```python
from build123d import *

# Parameters (mm, degrees)
SKETCH_22_W         = 80
SKETCH_22_H         = 80
SKETCH_22_R         = 1.6
SKETCH_22_R_2       = 23.7
SKETCH_22_R_3       = 2.6
EXTRUDE_1_DEPTH     = 15
SKETCH_24_R         = 2.9
CUT_EXTRUDE_2_DEPTH = 5
SKETCH_26_R         = 4.5
CUT_EXTRUDE_4_DEPTH = 5
SKETCH_31_R         = 1.8
CUT_EXTRUDE_6_DEPTH = 12
SKETCH_36_R         = 1.8
CUT_EXTRUDE_9_DEPTH = 12


with BuildPart() as part:
    # 草图22 → 凸台-拉伸1 (new body)
    with BuildSketch(Plane(origin=(0, 0, 0), x_dir=(1, 0, 0), z_dir=(0, 1, 0))):
        Rectangle(SKETCH_22_W, SKETCH_22_H)
        with Locations((0, 37)):
            Circle(SKETCH_22_R, mode=Mode.SUBTRACT)
        with Locations((26.162950904, 26.162950904)):
            Circle(SKETCH_22_R, mode=Mode.SUBTRACT)
        with Locations((37, 0)):
            Circle(SKETCH_22_R, mode=Mode.SUBTRACT)
        with Locations((26.162950904, -26.162950904)):
            Circle(SKETCH_22_R, mode=Mode.SUBTRACT)
        with Locations((0, -37)):
            Circle(SKETCH_22_R, mode=Mode.SUBTRACT)
        with Locations((-26.162950904, -26.162950904)):
            Circle(SKETCH_22_R, mode=Mode.SUBTRACT)
        with Locations((-37, 0)):
            Circle(SKETCH_22_R, mode=Mode.SUBTRACT)
        with Locations((-26.162950904, 26.162950904)):
            Circle(SKETCH_22_R, mode=Mode.SUBTRACT)
        Circle(SKETCH_22_R_2, mode=Mode.SUBTRACT)
        with Locations((-31.819805153, 31.819805153)):
            Circle(SKETCH_22_R_3, mode=Mode.SUBTRACT)
        with Locations((-31.819805153, -31.819805153)):
            Circle(SKETCH_22_R_3, mode=Mode.SUBTRACT)
        with Locations((31.819805153, -31.819805153)):
            Circle(SKETCH_22_R_3, mode=Mode.SUBTRACT)
        with Locations((31.819805153, 31.819805153)):
            Circle(SKETCH_22_R_3, mode=Mode.SUBTRACT)
    extrude(amount=EXTRUDE_1_DEPTH)

    # 草图24 → 切除-拉伸2 (cut)
    with BuildSketch(Plane.XZ):
        with Locations((0, 37)):
            Circle(SKETCH_24_R)
        with Locations((26.162950904, 26.162950904)):
            Circle(SKETCH_24_R)
        with Locations((37, 0)):
            Circle(SKETCH_24_R)
        with Locations((26.162950904, -26.162950904)):
            Circle(SKETCH_24_R)
        with Locations((0, -37)):
            Circle(SKETCH_24_R)
        with Locations((-26.162950904, -26.162950904)):
            Circle(SKETCH_24_R)
        with Locations((-37, 0)):
            Circle(SKETCH_24_R)
        with Locations((-26.162950904, 26.162950904)):
            Circle(SKETCH_24_R)
    extrude(amount=-CUT_EXTRUDE_2_DEPTH, mode=Mode.SUBTRACT)

    # 草图26 → 切除-拉伸4 (cut)
    with BuildSketch(Plane(origin=(0, 15, 0), x_dir=(1, 0, 0), z_dir=(0, 1, 0))):
        with Locations((-31.819805153, 31.819805153)):
            Circle(SKETCH_26_R)
        with Locations((31.819805153, 31.819805153)):
            Circle(SKETCH_26_R)
        with Locations((31.819805153, -31.819805153)):
            Circle(SKETCH_26_R)
        with Locations((-31.819805153, -31.819805153)):
            Circle(SKETCH_26_R)
    extrude(amount=-CUT_EXTRUDE_4_DEPTH, mode=Mode.SUBTRACT)

    # 草图31 → 切除-拉伸6 (cut)
    with BuildSketch(Plane.XY.offset(40)):
        with Locations((13.998307963, 7.310553575)):
            Circle(SKETCH_31_R)
    extrude(amount=-CUT_EXTRUDE_6_DEPTH, mode=Mode.SUBTRACT)

    # 草图36 → 切除-拉伸9 (cut)
    with BuildSketch(Plane(origin=(0, 0, -40), x_dir=(-1, 0, 0), z_dir=(0, 0, -1))):
        with Locations((-16.504769552, 7.351157317)):
            Circle(SKETCH_36_R)
    extrude(amount=-CUT_EXTRUDE_9_DEPTH, mode=Mode.SUBTRACT)


solid = part.part
```
Could you check a few things on this model? Use its own coordinates, in mm. A direction names the side the tool comes from. Coordinates: 2 decimals unless noted, no trailing zeros. Order: outer loops, then holes, each group sorted by start corner. A loop starts at its lowest first (then second) coordinate and runs counter-clockwise, first axis right, second up. Notation, with made-up numbers: M 55,-35.5 L 61,-35.5 A21 cw 61,-16.5 Z; hole C -26.75,52 d7. An arc over 180 degrees is marked long. Use a Markdown table: item, result. Add a question column.
Q1. Which directions (+Z, -Z, +X, -X, +Y, -Y) give clear straight access to the entire face, cutting with the end or side of a thin tool? Please do faces 5 (the cylindrical face through (-25.3, 9.93, -27.51)), 6 (the flat face through (27.41, 5, -27.41)), 7 (the cylindrical face through (14.842, 6.662, -34.084)), 8 (the flat face through (-1, 7, 40)), 9 (the cylindrical face through (-36.315, 12.535, 31.622)).
Q2. I'm going to push a flat-ended pin straight in: pin 1 (3.5 mm diameter, centred on x = 0, z = 37, fed in from -Y). Where does the tip first touch, or does it pass through?
Q3. I want a section at C-C on y = 11.25. Give the number of separate pieces and of enclosed holes in the cut face, then the cut area to 3 significant figures.
Q4. I want a section at D-D on z = 15. List the corners of the cut face in (x, y) for me, then the cut area to 3 significant figures.
Q5. If I drill on L1, parallel to X at y = 12.75, z = 0; L2, parallel to Z at x = -37, y = 12.5, over which ranges is the centre line in solid material (lowest first)?
Q6. We'd pull the mould along Z, two halves only. Please class faces 1 (the cylindrical face through (-38.18, 9.93, -1.08)), 2 (the cylindrical face through (12.57, 6.215, 34.084)), 3 (the flat face through (17, 7, -28)), 4 (the cylindrical face through (-29.34, 4.93, 31.04)): pulls with the +Z half, pulls with the -Z half, needs draft (parallel to the pull), parting line crosses it, or undercut.
Q7. I want a section at B-B on x = 0. List the corners of the cut face in (y, z) for me, then the cut area to 3 significant figures.
Q8. I want a section at A-A on z = 0. List the corners of the cut face in (x, y) for me, then the cut area to 3 significant figures.
Checked values:
| question | item | result |
|---|---|---|
| 1 | face 5 | +Y, -Y |
| 1 | face 6 | -Y |
| 1 | face 7 | -Z |
| 1 | face 8 | +Z, +X, -X, +Y, -Y |
| 1 | face 9 | +Y |
| 2 | pin 1 | y = 5 |
| 3 | separate pieces | 1 |
| 3 | enclosed holes | 13 |
| 3 | area | 4,320 mm² |
| 4 | outline | M -40,0 L -18.35,0 L -18.35,15 L -40,15 Z; M 18.35,0 L 40,0 L 40,15 L 18.35,15 Z |
| 4 | area | 650 mm² |
| 5 | L1 | -40 to -38.6, -35.4 to -23.7, 23.7 to 35.4, 38.6 to 40 |
| 5 | L2 | -40 to -1.6, 1.6 to 40 |
| 6 | face 1 | undercut |
| 6 | face 2 | needs draft |
| 6 | face 3 | pulls with the -Z half |
| 6 | face 4 | undercut |
| 7 | outline | M 0,-40 L 15,-40 L 15,-38.6 L 5,-38.6 L 5,-39.9 L 0,-39.9 Z; M 0,-34.1 L 5,-34.1 L 5,-35.4 L 15,-35.4 L 15,-23.7 L 0,-23.7 Z; M 0,23.7 L 15,23.7 L 15,35.4 L 5,35.4 L 5,34.1 L 0,34.1 Z; M 0,39.9 L 5,39.9 L 5,38.6 L 15,38.6 L 15,40 L 0,40 Z |
| 7 | area | 367 mm² |
| 8 | outline | M -40,0 L -39.9,0 L -39.9,5 L -38.6,5 L -38.6,15 L -40,15 Z; M -35.4,5 L -34.1,5 L -34.1,0 L -23.7,0 L -23.7,15 L -35.4,15 Z; M 23.7,0 L 34.1,0 L 34.1,5 L 35.4,5 L 35.4,15 L 23.7,15 Z; M 38.6,5 L 39.9,5 L 39.9,0 L 40,0 L 40,15 L 38.6,15 Z |
| 8 | area | 367 mm² |
